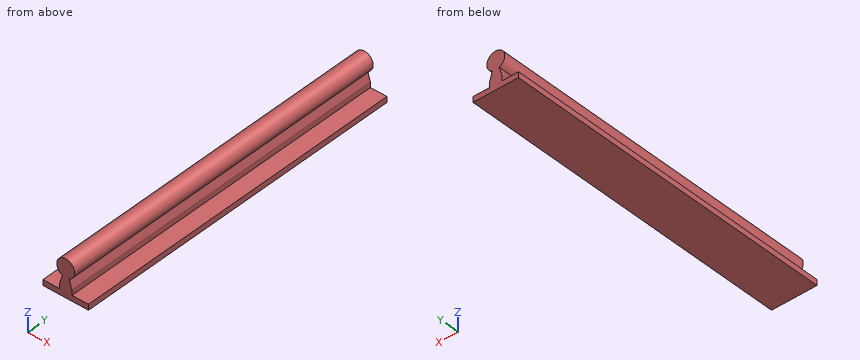
```python
from build123d import *

# Parameters (mm, degrees)
F1_DEPTH = 300


with BuildPart() as f1:
    # F0 (on Front) → F1 (new body)
    with BuildSketch(Plane.XZ):
        with BuildLine():
            Line((5.400592, -15.418472), (3.027247, -7.405118))
            ThreePointArc((3.027247, -7.405118), (0, 8), (-3.027247, -7.405118))
            Line((-3.027247, -7.405118), (-5.400592, -15.418472))
            Line((-5.400592, -15.418472), (-5.400592, -20.151161))
            Line((-5.400592, -20.151161), (-20.206842, -20))
            Line((-20.206842, -20), (-20.206842, -25))
            Line((-20.206842, -25), (0, -25))
            Line((0, -25), (20.2184, -25))
            Line((20.2184, -25), (20.2184, -19.999882))
            Line((20.2184, -19.999882), (5.400592, -20.151161))
            Line((5.400592, -20.151161), (5.400592, -15.418472))
        make_face()
    extrude(amount=F1_DEPTH)


solid = f1.part
```
Can you work these out from the model? Positions are in its coordinate system, mm. Round coordinates to 2 decimals unless told otherwise and drop trailing zeros. Order: outer loops, then holes, each group sorted by start corner. A loop starts at its lowest first (then second) coordinate and runs counter-clockwise, first axis right, second up.
(1) I'm going to push flat-ended pins straight in: pin 1 (5 mm diameter, centred on y = -209.5, z = -17, fed in from -X); pin 2 (4 mm diameter, centred on y = -186, z = -18.5, fed in from +X); pin 3 (5 mm diameter, centred on y = -68, z = -16.5, fed in from +X); pin 4 (8 mm diameter, centred on x = -10.5, y = -109, fed in from +Z). Where does each tip first touch, or does it pass through?
Results are:
pin 1: stops at x = -5.4
pin 2: stops at x = 20.22
pin 3: stops at x = 5.4
pin 4: stops at z = 4.66
(2) If we section it at C-C (x = -15): Please give me the cut outline in (y, z).
Results are:
outline: (-300, -25) - (0, -25) - (0, -20.05) - (-300, -20.05) - close
(3) If we section it at A-A (y = -64.5): Please give me the cut outline in (x, z), plus the area to 3 significant figures.
Results are:
outline: (-20.21, -25) - (20.22, -25) - (20.22, -20) - (5.4, -20.15) - (5.4, -15.42) - (3.03, -7.41) arc R8 ccw (long way) to (-3.03, -7.41) - (-5.4, -15.42) - (-5.4, -20.15) - (-20.21, -20) - close
area: 516 mm2
(4) If we section it at B-B (z = 0): Please give me the cut outline in (x, y).
Results are:
outline: (-8, -300) - (8, -300) - (8, 0) - (-8, 0) - close
(5) If I drill on L1, parallel to Z at x = -9, y = -249; L2, parallel to Z at x = 17, y = -172; L3, parallel to X at y = -38.5, z = 0.5, over which ranges is the centre line in solid material (lowest first)?
Results are:
L1: z = -25 to -20.11
L2: z = -25 to -20.03
L3: x = -7.98 to 7.98
